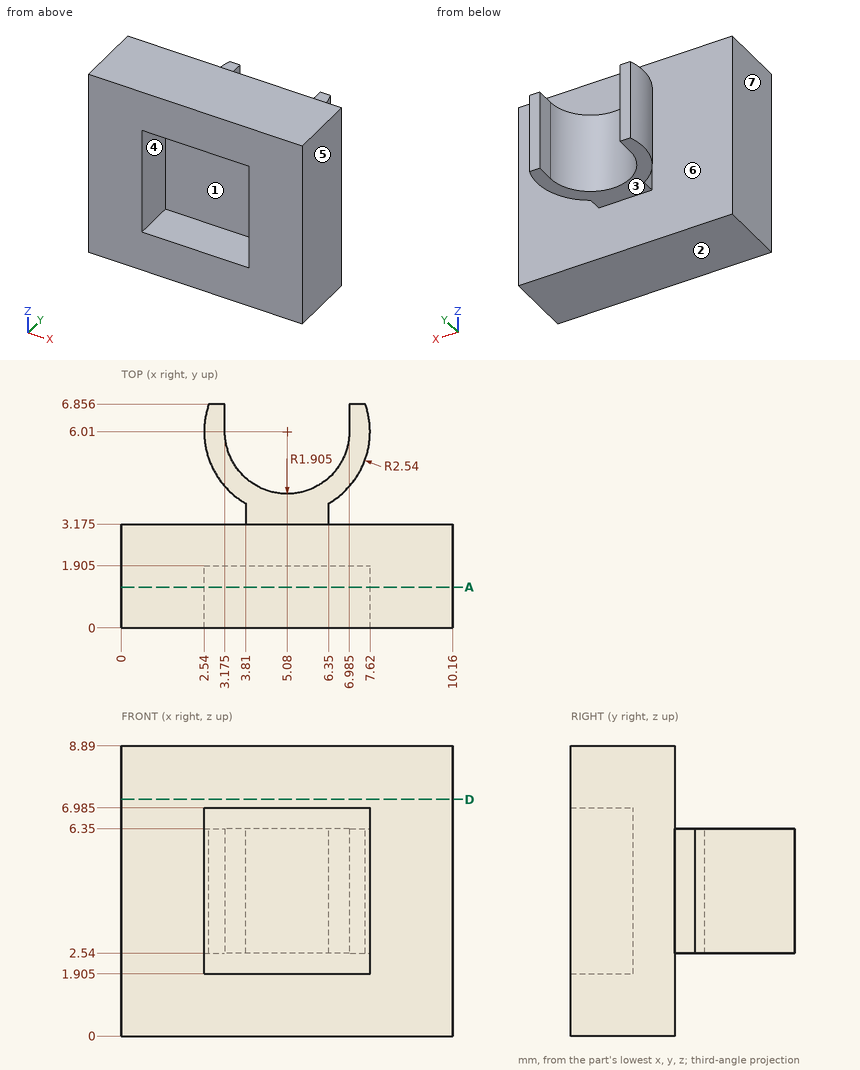
Geometry: see drawing. Coordinates: mm, zero at the bounding-box minimum. A direction names the side the tool comes from. Round coordinates to 2 decimals unless told otherwise and drop trailing zeros. Loops run counter-clockwise (first coordinate to the right, second up) from the corner with the lowest first, then second, coordinate; pieces in that order, holes last.
(1) Section query D-D (z = 7.25). Output: boundary loops of the cut face in (x, y) (1 decimal).
From the geometry:
outline: (0, 0) - (10.2, 0) - (10.2, 3.2) - (0, 3.2) - close
(2) Section query A-A (y = 1.25). Output: boundary loops of the cut face in (x, z) (1 decimal).
From the geometry:
outline: (0, 0) - (10.2, 0) - (10.2, 8.9) - (0, 8.9) - close; hole (2.5, 1.9) - (7.6, 1.9) - (7.6, 7) - (2.5, 7) - close
(3) Contact query for flat-ended pins moving along their axis: pin 1 Ø0.9 at (y, z) = (6.5, 4) entering from -X; pin 2 Ø1.1 at (x, y) = (6, 4) entering from -Z; pin 3 Ø1.1 at (x, y) = (6, 5.5) entering from +Z; pin 4 Ø2.5 at (x, z) = (4, 4.5) entering from -Y (3 decimals). Output: stop coordinate, or through.
From the geometry:
pin 1: stops at x = 2.54
pin 2: stops at z = 2.54
pin 3: passes through
pin 4: stops at y = 1.905
(4) Material intervals for probe 1 along Z at (x, y) = (5.75, 1) (1 decimal); probe 2 along X at (y, z) = (0.5, 3.5); probe 3 along Y at (x, z) = (2, 6.75) (1 decimal), sorted ascending.
From the geometry:
probe 1: z = 0 to 1.9, 7 to 8.9
probe 2: x = 0 to 2.54, 7.62 to 10.16
probe 3: y = 0 to 3.2
(5) Pull-direction query (X, two-part tool) for the marked faces 4, 5, 6 and 7; classes: +X half, -X half, draft (parallel to the pull), parting line (faces both ways), or undercut.
From the geometry:
face 4: undercut
face 5: +X half
face 6: draft
face 7: -X half
(6) Access query for the marked faces 1, 2 and 3. Directions: +Z, -Z, +X, -X, +Y, -Y. A direction counts if a zero-diameter tool reaches every point of the face in a straight line with its end or side. Return the directions, or none.
From the geometry:
face 1: -Y
face 2: -Z, +X, -X, +Y, -Y
face 3: -Z, +X, -X, +Y
